Autodesk Inventor part; units mm, degrees
ref_plane "YZ Plane" through (0, 0, 0) normal (1, 0, 0) x (0, 1, 0)
ref_plane "XZ Plane" through (0, 0, 0) normal (0, 1, 0) x (-1, 0, 0)
ref_plane "XY Plane" through (0, 0, 0) normal (0, 0, 1) x (1, 0, 0)
sketch "Sketch1" plane through (0, 0, 0) normal (0, 0, 1) x (1, 0, 0)
  line L0 (0, 0) -> (34.3335, 0)
  line L1 (33.676, 1.5875) -> (0, 1.5875)
  line L2 (0, 1.5875) -> (0, 0)
  line L3 (34.3335, 0) -> (254, 219.6665)
  line L4 (1.1112, 2.6987) -> (251.3012, 252.8888)
  line L5 (33.676, 1.5875) -> (252.4125, 220.324)
  line L6 (1.1112, 2.6987) -> (32.0885, 2.6988)
  arc A0 (32.0885, 1.5875) -> (32.0885, 2.6988) centre (32.0885, 2.1431) ccw
  line L7 (252.4125, 220.324) -> (252.4125, 254)
  line L8 (252.4125, 254) -> (254, 254)
  line L9 (254, 254) -> (254, 219.6665)
  line L10 (251.3012, 252.8888) -> (251.3012, 221.9115)
  arc A1 (251.3012, 221.9115) -> (252.4125, 221.9115) centre (251.8569, 221.9115) ccw
  dimension "d0" = 25.4
  dimension "d1" = 135
  dimension "d2" = 1.5875
  dimension "d3" = 1.5875
  dimension "d4" = 1.1113
  dimension "d5" = 1.5875
  dimension "d6" = 1.5875
  dimension "d7" = 254
  dimension "d9" = 1.1113
  dimension "d10" = 1.5875
extrude "Extrusion1" add sketch "Sketch1" along normal blind 1.5875 contours A0 L6 L4 L10 A1 L7 L5 L1
extrude "Extrusion2" add sketch "Sketch1" along normal blind 25.4 contours L2 L1 L5 L7 L8 L9 L3 L0
equation "\"d3\" = d2"
equation "\"d4\" = 0.7 * d2"
equation "\"d5\" = d2"
equation "\"d6\" = d2"
equation "\"d9\" = d4"
equation "\"d10\" = d6"
properties part number "electronics board support outside"
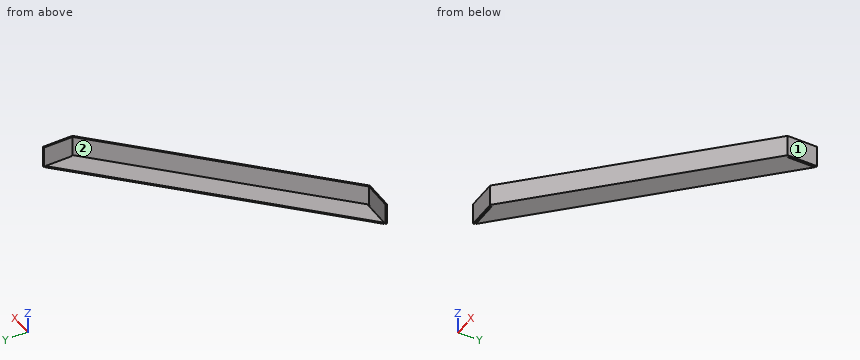
Geometry: final body of the model. Coordinates: model frame, mm. Face numbers are marked on the shaded views. A direction names the side the tool comes from. Coordinates: 2 decimals unless noted, no trailing zeros. Order: outer loops, then holes, each group sorted by start corner. A loop starts at its lowest first (then second) coordinate and runs counter-clockwise, first axis right, second up.
1) Section D-D (y = 192.5). Return loops of the section in (x, z).
Result sheet:
outline: (190.91, 0) - (226.83, 0) - (226.83, 25.4) - (224.59, 25.4) - (224.59, 1.59) - (190.91, 1.59) - close
2) Ray query, probe 1 along X at (y, z) = (239, 19); probe 2 along X at (y, z) = (93.5, 14.5); probe 3 along Y at (x, z) = (138.5, 15.5). Return the intervals inside material, ascending.
Result sheet:
probe 1: x = 252.41 to 254
probe 2: x = 125.59 to 127.83
probe 3: y = 104.17 to 106.41
3) Set-up query: the marked faces 1 and 2. Return all of +Z, -Z, +X, -X, +Y, -Y with unobstructed straight access to the full face (end or side cutting, diameter ignored); none if empty.
Result sheet:
face 1: +Z, -Z, +X, +Y, -Y
face 2: +Z, -X, +Y
4) Section A-A (z = 6). Return loops of the section in (x, y).
Result sheet:
outline: (0, 0) - (34.33, 0) - (254, 219.67) - (254, 254) - (252.41, 254) - (252.41, 220.32) - (33.68, 1.59) - (0, 1.59) - close
5) Section B-B (y = 237). Return loops of the section in (x, z), then the cut area to 3 significant figures.
Result sheet:
outline: (235.41, 0) - (251.3, 0) - (251.3, 1.59) - (235.41, 1.59) - close; (252.41, 0) - (254, 0) - (254, 25.4) - (252.41, 25.4) - close
area: 65.5 mm2
6) First-contact query: P1, Ø1.5, axis at y = 59.5, z = 11.5, coming from the -X side; P2, Ø3, axis at x = 27, z = 18, coming from the +Y side; P3, Ø12, axis at y = 90.5, z = 8.5, coming from the +X side. Flat tips, straight axial feed; report the tip coordinate or a pass-through.
Result sheet:
P1: stops at x = 90.84
P2: stops at y = 1.59
P3: stops at x = 130.83
7) Section C-C (x = 112). Return loops of the section in (y, z), then the cut area to 3 significant figures.
Result sheet:
outline: (77.67, 0) - (113.59, 0) - (113.59, 1.59) - (79.91, 1.59) - (79.91, 25.4) - (77.67, 25.4) - close
area: 110 mm2
